Check sheet for the modelled part. Datum: model origin and axes. Units: mm. A direction names the side the tool comes from. Coordinates: 2 decimals unless noted, no trailing zeros. Loops run counter-clockwise (first coordinate to the right, second up) from the corner with the lowest first, then second, coordinate; pieces in that order, holes last. Notation, with made-up numbers: M 4.5,38 L 31.5,38 A26 ccw 31.5,55 Z; hole C 34.5,81.25 d6. An arc over 180 degrees is marked long. Answer in a Markdown table with one row per item. Add a question column.
```python
from build123d import *

# Parameters (mm, degrees)
F1_DEPTH = 12
F2_T     = -1.5
F3_R     = 1
F4_DEPTH = 70
F5_W     = 18
F5_H     = 52.2
F6_DEPTH = 25
F9_DEPTH = 10.5


with BuildPart() as f1:
    # F0 (on Top) → F1 (new body)
    with BuildSketch(Plane.XY):
        Polygon((53.5, 32.5), (0, 32.5), (-53.5, 32.5), (-53.5, 17.5), (-46.5, 17.5), (-46.5, 0), (-46.5, -17.5), (-53.5, -17.5), (-53.5, -32.5), (0, -32.5), (53.5, -32.5), (53.5, -17.5), (46.5, -17.5), (46.5, 0), (46.5, 17.5), (53.5, 17.5), align=None)
    extrude(amount=F1_DEPTH)

    # F2
    f2_openings = [f1.faces().sort_by_distance(p)[0] for p in [
        (0, 0, 12),
    ]]
    offset(amount=F2_T, openings=f2_openings)

    # F3 (on face) → F4 (cut)
    with BuildSketch(Plane.XZ.offset(32.5)):
        with Locations((0, 2.5)):
            Circle(F3_R)
    extrude(amount=-F4_DEPTH, mode=Mode.SUBTRACT)

    # F5 (on face) → F6 (cut)
    with BuildSketch(Plane(origin=(0, 0, 0), x_dir=(1, 0, 0), z_dir=(0, 0, -1))):
        Polygon((-19.9, 26.1), (-46.5, 26.1), (-46.5, 17.5), (-46.5, -17.5), (-46.5, -26.1), (-19.9, -26.1), align=None)
        Rectangle(F5_W, F5_H)
        Polygon((46.5, -17.5), (46.5, 17.5), (46.5, 26.1), (19.9, 26.1), (19.9, -26.1), (46.5, -26.1), align=None)
    extrude(amount=-F6_DEPTH, mode=Mode.SUBTRACT)

    # F8 (on face) → F9 (join)
    with BuildSketch(Plane.XY.offset(1.5)):
        Polygon((-19.9, 17.5), (-12.9, 17.5), (-12.9, 31), (-14.362971, 31), (-14.362971, 19), (-19.9, 19), align=None)
        Polygon((12.9, 31), (12.9, 17.5), (19.9, 17.5), (19.9, 19), (14.362971, 19), (14.362971, 31), align=None)
        Polygon((19.9, -17.5), (12.9, -17.5), (12.9, -31), (14.362971, -31), (14.362971, -19), (19.9, -19), align=None)
        Polygon((-19.9, -17.5), (-19.9, -19), (-14.362971, -19), (-14.362971, -31), (-12.9, -31), (-12.9, -17.5), align=None)
    extrude(amount=F9_DEPTH)


solid = f1.part
```
Q1. Go/stop test with a flat-tipped pin: pin 1 (3 mm diameter, centred on x = -22, y = -24, fed in from -Z). Record where the tip stops, or that it passes through.
Q2. Cross-section at B-B (x = 3). Record the cut outline in (y, z), plus the area to 3 significant figures.
Q3. Thickness scan on L1, parallel to X at y = 23.5, z = 3.5; L2, parallel to Y at x = -28, z = 11.5; L3, parallel to X at y = 31.7, z = 2.5. Record the ranges inside material, lowest first.
Q4. Access from +Z, -Z, +X, -X, +Y, -Y to the whole of each face (thin tool, end or side, straight path). Record for faces 5 (the face through (46.5, -18.6, 4.2)), 6 (the face through (-33, -31, 7)), 7 (the face through (-16, -17.5, 7)), 8 (the face through (-1, -32.5, 6)).
Q5. Mould release check, pull along X, two halves, no side actions. Record for faces 1 (the face through (-17, 19, 7)), 2 (the face through (50, 17.5, 6)), 3 (the face through (-53.5, 25, 6)), 4 (the face through (0, 31, 7)): released by +X, released by -X, zero draft, split by the parting line, or undercut.
Q6. Cross-section at A-A (y = -21.5). Record the cut outline in (x, z).
Answer key:
| question | item | result |
|---|---|---|
| 1 | pin 1 | through |
| 2 | outline | M -32.5,0 L -26.1,0 L -26.1,1.5 L -31,1.5 L -31,12 L -32.5,12 Z; M 26.1,0 L 32.5,0 L 32.5,12 L 31,12 L 31,1.5 L 26.1,1.5 Z |
| 2 | area | 50.7 mm^2 |
| 3 | L1 | -53.5 to -52, -14.36 to -12.9, 12.9 to 14.36, 52 to 53.5 |
| 3 | L2 | -32.5 to -31, 31 to 32.5 |
| 3 | L3 | -53.5 to -1, 1 to 53.5 |
| 4 | face 5 | +Z, -Z |
| 4 | face 6 | +Z |
| 4 | face 7 | +Z, +X, -X |
| 4 | face 8 | +Z, -Z, +X, -X, -Y |
| 5 | face 1 | undercut |
| 5 | face 2 | zero draft |
| 5 | face 3 | released by -X |
| 5 | face 4 | undercut |
| 6 | outline | M -53.5,0 L -46.5,0 L -46.5,1.5 L -52,1.5 L -52,12 L -53.5,12 Z; M -19.9,0 L -9,0 L -9,1.5 L -12.9,1.5 L -12.9,12 L -14.36,12 L -14.36,1.5 L -19.9,1.5 Z; M 9,0 L 19.9,0 L 19.9,1.5 L 14.36,1.5 L 14.36,12 L 12.9,12 L 12.9,1.5 L 9,1.5 Z; M 46.5,0 L 53.5,0 L 53.5,12 L 52,12 L 52,1.5 L 46.5,1.5 Z |
